Can you work these out from the model? Positions are in its coordinate system, mm. A direction names the side the tool comes from. Give positions to 0.01 mm unless a question says otherwise; leave off trailing zeros. Loops run counter-clockwise (first coordinate to the right, second up) from the corner with the lowest first, then second, coordinate; pieces in that order, holes last. Notation, with made-up numbers: (-19, 27.5) - (29, 27.5) arc R9 ccw to (29, 32.5) - close; hole circle Ø6 at (-9, 56). An arc over 180 degrees is marked (long way). Write item = value, one per line.
Autodesk Inventor part; units mm, degrees
ref_plane "YZ Plane" through (0, 0, 0) normal (1, 0, 0) x (0, 1, 0)
ref_plane "XZ Plane" through (0, 0, 0) normal (0, 1, 0) x (-1, 0, 0)
ref_plane "XY Plane" through (0, 0, 0) normal (0, 0, 1) x (1, 0, 0)
sketch "Sketch1" plane through (0, 0, 0) normal (0, 1, 0) x (-1, 0, 0)
  circle A0 centre (0, 0) radius 32.385
  circle A1 centre (0, 0) radius 38.1
  line L0 (0, 38.1) -> (0, 32.385)
  line L1 (0, -32.385) -> (0, -38.1)
  dimension "d0" = 64.77
  dimension "d1" = 76.2
extrude "Extrusion1" add sketch "Sketch1" along normal blind 76.2 contours A0 L1 A1 L0 picked at (-2.826, -35.8766)
sketch "Sketch2" plane through (0, 76.2, 0) normal (0, 1, 0) x (1, 0, 0)
  arc A0 (0, -32.385) -> (0, 32.385) centre (0, 0) ccw
  line L0 (32.385, 0) -> (70.485, 0)
  line L1 (70.485, 0) -> (70.485, -25.4)
  line L2 (70.485, -25.4) -> (28.3981, -25.4)
  arc A1 (0, -38.1) -> (0, 38.1) centre (0, 0) ccw
  line L3 (70.485, 0) -> (70.485, 25.4)
  line L4 (70.485, 25.4) -> (28.3981, 25.4)
  arc A2 (28.3981, -25.4) -> (28.3981, 25.4) centre (0, 0) ccw
  dimension "d4" = 38.1
  dimension "d5" = 25.4
  dimension "d6" = 25.4
extrude "Extrusion2" add sketch "Sketch2" against normal blind 76.2
sketch "Sketch3" plane through (0, 76.2, 0) normal (0, 1, 0) x (1, 0, 0)
  line L0 (70.485, -25.4) -> (28.3981, -25.4)
  line L1 (70.485, -25.4) -> (64.135, -25.4)
  line L2 (64.135, -25.4) -> (64.135, -38.1)
  line L3 (64.135, -38.1) -> (70.485, -38.1)
  line L4 (70.485, -38.1) -> (70.485, -25.4)
  line L5 (28.3981, 25.4) -> (70.485, 25.4)
  line L6 (70.485, 25.4) -> (64.135, 25.4)
  line L7 (64.135, 25.4) -> (64.135, 38.1)
  line L8 (64.135, 38.1) -> (70.485, 38.1)
  line L9 (70.485, 38.1) -> (70.485, 25.4)
  point P0 (0, 0)
  dimension "d9" = 6.35
  dimension "d10" = 12.7
  dimension "d11" = 6.35
  dimension "d12" = 12.7
extrude "Extrusion3" add sketch "Sketch3" against normal blind 76.2
sketch "Sketch4" plane through (70.485, 76.2, 38.1) normal (1, 0, 0) x (0, 0, -1)
  line L0 (0, -76.2) -> (0, 0)
  line L1 (0, 0) -> (12.7, 0)
  line L2 (12.7, 0) -> (12.7, -76.2)
  line L3 (12.7, -76.2) -> (0, -76.2)
  line L4 (0, -76.2) -> (0, 0)
  line L5 (63.5, 0) -> (63.5, -76.2)
  line L6 (76.2, 0) -> (76.2, -76.2)
  line L7 (63.5, -76.2) -> (76.2, -76.2)
  line L8 (76.2, -76.2) -> (76.2, 0)
  line L9 (76.2, 0) -> (63.5, 0)
  line L10 (63.5, 0) -> (63.5, -76.2)
  line L11 (0, -76.2) -> (12.7, -76.2)
  line L12 (12.7, -76.2) -> (12.7, -63.5)
  line L13 (12.7, -63.5) -> (0, -63.5)
  line L14 (0, -63.5) -> (0, -76.2)
  line L15 (0, 0) -> (76.2, 0)
  line L16 (0, 0) -> (12.7, 0)
  line L17 (12.7, 0) -> (12.7, -12.7)
  line L18 (12.7, -12.7) -> (0, -12.7)
  line L19 (0, -12.7) -> (0, 0)
  line L20 (63.5, -76.2) -> (76.2, -76.2)
  line L21 (76.2, -76.2) -> (76.2, -63.5)
  line L22 (76.2, -63.5) -> (63.5, -63.5)
  line L23 (63.5, -63.5) -> (63.5, -76.2)
  line L24 (63.5, 0) -> (76.2, 0)
  line L25 (76.2, 0) -> (76.2, -12.7)
  line L26 (76.2, -12.7) -> (63.5, -12.7)
  line L27 (63.5, -12.7) -> (63.5, 0)
  point P0 (38.1, -76.2)
  dimension "d15" = 12.7
  dimension "d16" = 12.7
  dimension "d17" = 12.7
  dimension "d18" = 12.7
  dimension "d19" = 12.7
  dimension "d20" = 12.7
  dimension "d21" = 12.7
  dimension "d22" = 12.7
extrude "Extrusion4" cut sketch "Sketch4" against normal blind 36.5125 contours L0 L18 L2 L13 | L26 L6 L22 L5
sketch "Sketch5" plane through (70.485, 76.2, 38.1) normal (1, 0, 0) x (0, 0, -1)
  line L0 (12.7, -12.7) -> (0, -12.7)
  line L1 (0, -76.2) -> (0, 0)
  line L2 (12.7, -12.7) -> (0, -12.7)
  line L3 (0, -12.7) -> (0, 0)
  line L4 (0, 0) -> (12.7, 0)
  line L5 (12.7, 0) -> (12.7, -12.7)
  line L6 (76.2, -12.7) -> (63.5, -12.7)
  line L7 (63.5, 0) -> (76.2, 0)
  line L8 (63.5, -12.7) -> (76.2, -12.7)
  line L9 (76.2, -12.7) -> (76.2, 0)
  line L10 (76.2, 0) -> (63.5, 0)
  line L11 (63.5, 0) -> (63.5, -12.7)
  line L12 (12.7, -63.5) -> (0, -63.5)
  line L13 (0, -76.2) -> (12.7, -76.2)
  line L14 (12.7, -63.5) -> (0, -63.5)
  line L15 (0, -63.5) -> (0, -76.2)
  line L16 (0, -76.2) -> (12.7, -76.2)
  line L17 (12.7, -76.2) -> (12.7, -63.5)
  line L18 (63.5, -63.5) -> (63.5, -12.7)
  line L19 (63.5, -76.2) -> (76.2, -76.2)
  line L20 (63.5, -63.5) -> (76.2, -63.5)
  line L21 (76.2, -63.5) -> (76.2, -76.2)
  line L22 (76.2, -76.2) -> (63.5, -76.2)
  line L23 (63.5, -76.2) -> (63.5, -63.5)
  circle A0 centre (6.35, -6.35) radius 2.25
  circle A1 centre (69.85, -6.35) radius 2.25
  circle A2 centre (6.35, -69.85) radius 2.25
  circle A3 centre (69.85, -69.85) radius 2.25
  point P0 (38.1, -76.2)
  dimension "d25" = 4.5
  dimension "d26" = 4.5
  dimension "d27" = 4.5
  dimension "d28" = 4.5
extrude "Extrusion5" cut sketch "Sketch5" against normal blind 36.5125 contours A0 | A1 | A2 | A3
thicken "Thicken1" operation add thickness 25.4 both sides no extend neighbours yes toward (0, -1, 0) faces at (53.473, 76.2, 1.3012)
properties part number "motor support"
Q1. Which directions (+Z, -Z, +X, -X, +Y, -Y) give clear straight access to the entire face, cutting with the end or side of a thin tool? Please do faces 4 (the cylindrical face through (67.35, 5.49, -33.83)), 5 (the flat face through (67, 12.7, 32)), 6 (the flat face through (67, 12.7, -32)), 7 (the cylindrical face through (15.35, 25.04, -34.87)).
Output:
face_4 = +X
face_5 = +Z, +X, +Y
face_6 = -Z, +X, +Y
face_7 = -Z, +Y, -Y
Q2. Imagine slicing it at A-A, the plane y = 6.35. Write out the boundary of the cut face in (x, z) (3 decimals), then the cut area to 3 significant figures.
Output:
outline = (0, -38.1) arc R38.1 ccw to (28.398, -25.4) - (64.135, -25.4) - (64.135, -29.5) - (70.485, -29.5) - (70.485, 29.5) - (64.135, 29.5) - (64.135, 25.4) - (28.398, 25.4) arc R38.1 ccw to (0, 38.1) - (0, 32.385) arc R32.385 cw to (0, -32.385) - close; (64.135, -38.1) - (70.485, -38.1) - (70.485, -34) - (64.135, -34) - close; (64.135, 34) - (70.485, 34) - (70.485, 38.1) - (64.135, 38.1) - close
area = 2,540 mm2
Q3. For pin 1 (3 mm diameter, centred on x = 32.5, y = 10, fed in from +Z); pin 2 (3 mm diameter, centred on x = 28, y = 24.5, fed in from -Z); pin 3 (7 mm diameter, centred on x = 67.5, z = -31, fed in from +Y), each with a flat end and sliding along its axis, tell me the tip position at first contact or that it passes through.
Output:
pin_1 = 25.4
pin_2 = -27.37
pin_3 = 12.7
Q4. Imagine slicing it at C-C, the plane y = 41.5. Write out the boundary of the cut face in (x, z) (3 decimals), then the cut area to 3 significant figures.
Output:
outline = (0, -38.1) arc R38.1 ccw to (28.398, -25.4) - (70.485, -25.4) - (70.485, 25.4) - (28.398, 25.4) arc R38.1 ccw to (0, 38.1) - (0, 32.385) arc R32.385 cw to (0, -32.385) - close
area = 2,430 mm2
Q5. Imagine slicing it at B-B, the plane z = 0. Write out the boundary of the cut face in (x, y) (3 decimals), then the cut area to 3 significant figures.
Output:
outline = (32.385, 0) - (70.485, 0) - (70.485, 50.8) - (32.385, 50.8) - close
area = 1,940 mm2
Q6. I need wall thicknesses on L1, parallel to Y at x = 66.75, z = -31.75; L2, parallel to Z at x = 66, y = 6; L3, parallel to X at y = 42.5, z = -0.5 (3 decimals). Which ranges of each line are inside material? Lowest first, please.
Output:
L1 = 0 to 4.1, 8.6 to 12.7
L2 = -38.1 to -33.97, -29.53 to 29.53, 33.97 to 38.1
L3 = 32.381 to 70.485
Q7. Imagine slicing it at D-D, the plane z = -9. Write out the boundary of the cut face in (x, y) (3 decimals).
Output:
outline = (31.109, 0) - (70.485, 0) - (70.485, 50.8) - (31.109, 50.8) - close
Q8. We'd pull the mould along X, two halves only. Please class faces 1 (the flat face through (64.135, 6, -29)), 2 (the cylindrical face through (67.354, 7.026, 29.604)), 3 (the flat face through (0, 25, -35)): released by +X, released by -X, zero draft, split by the parting line, or undercut.
Output:
face_1 = undercut
face_2 = zero draft
face_3 = released by -X
